```python
from build123d import *

# Parameters (mm, degrees)
BODY_DEPTH             = 88
SKETCH_2_W             = 30
SKETCH_2_H             = 1
CUT1_DEPTH             = 7.9
FIXTURE_M3_D           = 3.4
FIXTURE_M3_DEPTH       = 6
FIXTURE_M3_CBORE_D     = 6.5
FIXTURE_M3_CBORE_DEPTH = 3.4
FIXTURE_M3_TIP         = 1.021463052
PATTERN_LINEAR_1_COUNT = 4
PATTERN_LINEAR_1_PITCH = 20


with BuildPart() as part:
    # Эскиз1 → Body (new body)
    with BuildSketch(Plane.XY):
        Polygon((-15, -3), (15, -3), (15, 3), (15, 10.6), (13.3, 10.6), (13.3, 3), (4.5, 3), (4.5, 1.5), (-4.5, 1.5), (-4.5, 3), (-13.3, 3), (-13.3, 10.6), (-15, 10.6), (-15, 3), align=None)
    extrude(amount=BODY_DEPTH)

    # Эскиз2 → Cut1 (cut)
    with BuildSketch(Plane(origin=(0, 10.6, 0), x_dir=(1, 0, 0), z_dir=(0, 1, 0))):
        with Locations((0, -87.5)):
            Rectangle(SKETCH_2_W, SKETCH_2_H)
        with Locations((0, -0.5)):
            Rectangle(SKETCH_2_W, SKETCH_2_H)
    extrude(amount=-CUT1_DEPTH, mode=Mode.SUBTRACT)

    # Fixture M3
    with Locations(Plane(origin=(-8.5, 3, 71.5), x_dir=(1, 0, 0), z_dir=(0, 1, 0))):
        with Locations((0, 0), (17, 0), (17, 55), (0, 55)):
            CounterBoreHole(FIXTURE_M3_D / 2, FIXTURE_M3_CBORE_D / 2, FIXTURE_M3_CBORE_DEPTH, depth=FIXTURE_M3_DEPTH)
            with Locations((0, 0, -(FIXTURE_M3_DEPTH + FIXTURE_M3_TIP / 2))):  # 118° drill point
                Cone(0, FIXTURE_M3_D / 2, FIXTURE_M3_TIP, mode=Mode.SUBTRACT)

    # Эскиз7 → Fixture M2 (revolve, cut)
    with BuildSketch(Plane(origin=(0, 1.5, 73), x_dir=(0, 0, 1), z_dir=(1, 0, 0))):
        Polygon((0, 0), (0, 5.115882135), (1.025, 4.5), (1.025, 0), align=None)
    fixture_m2 = revolve(axis=Axis((0, 7.85, 73), (0, -1, 0)), mode=Mode.SUBTRACT)

    # Линейный массив1: Fixture M2 ×4
    with Locations(*[(0, 0, -i * PATTERN_LINEAR_1_PITCH) for i in range(1, PATTERN_LINEAR_1_COUNT)]):
        add(fixture_m2, mode=Mode.SUBTRACT)


solid = part.part
```
Input: part model. Units: mm. Frame: model coordinates. A direction names the side the tool comes from. Round coordinates to 2 decimals unless told otherwise and drop trailing zeros. Loops run counter-clockwise (first coordinate to the right, second up) from the corner with the lowest first, then second, coordinate; pieces in that order, holes last.
1) Section query C-C on y = -2. Count the separate pieces of the cut face and the enclosed holes in it, plus the area to 3 significant figures.
Ans:
separate pieces: 1
enclosed holes: 8
area: 2,590 mm2
2) Section query B-B on x = 8.5. Return the cut outline in (y, z).
Ans:
outline: (-3, 0) - (2.7, 0) - (2.7, 1) - (3, 1) - (3, 13.25) - (-0.4, 13.25) - (-0.4, 14.8) - (-3, 14.8) - close; (-3, 18.2) - (-0.4, 18.2) - (-0.4, 19.75) - (3, 19.75) - (3, 68.25) - (-0.4, 68.25) - (-0.4, 69.8) - (-3, 69.8) - close; (-3, 73.2) - (-0.4, 73.2) - (-0.4, 74.75) - (3, 74.75) - (3, 87) - (2.7, 87) - (2.7, 88) - (-3, 88) - close
3) Section query A-A on z = 53. Return the cut outline in (x, y) (3 decimals).
Ans:
outline: (-15, -3) - (-1.025, -3) - (-1.025, 1.5) - (-4.5, 1.5) - (-4.5, 3) - (-13.3, 3) - (-13.3, 10.6) - (-15, 10.6) - close; (1.025, -3) - (15, -3) - (15, 10.6) - (13.3, 10.6) - (13.3, 3) - (4.5, 3) - (4.5, 1.5) - (1.025, 1.5) - close
4) Section query D-D on y = 9. Return the cut outline in (x, z).
Ans:
outline: (-15, 1) - (-13.3, 1) - (-13.3, 87) - (-15, 87) - close; (13.3, 1) - (15, 1) - (15, 87) - (13.3, 87) - close
5) Pin query (flat end, axial travel): pin 1 (0.5 mm diameter, centred on x = 8, z = 0.5, fed in from +Y); pin 2 (2.5 mm diameter, centred on x = 0, z = 73, fed in from +Y); pin 3 (2 mm diameter, centred on x = -9.5, z = 18, fed in from +Y); pin 4 (4.5 mm diameter, centred on x = -8.5, z = 71.5, fed in from -Y). Return the tip coordinate at first contact, or that it passes through.
Ans:
pin 1: stops at y = 2.7
pin 2: stops at y = 1.5
pin 3: stops at y = -0.4
pin 4: stops at y = -3
6) Material intervals for line 1 (X direction, y = -2.2, z = 16.5); line 2 (Z direction, x = 0, y = -1.7) (3 decimals); line 3 (X direction, y = 2.35, z = 16.5), sorted ascending.
Ans:
line 1: x = -15 to -10.2, -6.8 to 6.8, 10.2 to 15
line 2: z = 0 to 11.975, 14.025 to 31.975, 34.025 to 51.975, 54.025 to 71.975, 74.025 to 88
line 3: x = -15 to -11.75, -5.25 to -4.5, 4.5 to 5.25, 11.75 to 15
7) Pull-direction query (Z, two-part tool) for faces 1 (the cylindrical face through (5.921, 1.324, 73.478)), 2 (the flat face through (0, 0, 88)), 3 (the flat face through (0, -3, 43)); classes: released by +Z, released by -Z, zero draft, split by the parting line, or undercut.
Ans:
face 1: undercut
face 2: released by +Z
face 3: zero draft
8) Set-up query: faces 4 (the flat face through (-14, 6, 1)), 5 (the flat face through (-14, 6, 87)), 6 (the flat face through (13.3, 7, 43)). Return all of +Z, -Z, +X, -X, +Y, -Y with unobstructed straight access to the full face (end or side cutting, diameter ignored); none if empty.
Ans:
face 4: -Z, +X, -X, +Y
face 5: +Z, +X, -X, +Y
face 6: +Z, -Z, +Y
